The listing builds one solid part. Answer for the finished solid, in the listing's coordinates (mm). Coordinates: 2 decimals unless noted, no trailing zeros. Order: outer loops, then holes, each group sorted by start corner. A loop starts at its lowest first (then second) coordinate and runs counter-clockwise, first axis right, second up. Notation, with made-up numbers: (-23, 3) - (7, 3) arc R16 ccw to (7, 28) - close; hole circle Ø7 at (11.25, 28.25). An arc over 180 degrees is marked (long way). One line per item, written item: value. Start each with the question number.
```python
from build123d import *

# Parameters (mm, degrees)
BOSS_EXTRUDE1_DEPTH             = 16
SKETCH2_W                       = 34
SKETCH2_H                       = 8
CUT_EXTRUDE1_DEPTH              = 0.5
SKETCH7_R                       = 8.5
CUT_EXTRUDE2_DEPTH              = 2
BOSS_EXTRUDE2_DEPTH             = 3
BOSS_EXTRUDE3_REACH             = 31.159
BOSS_EXTRUDE3_DIRECTION_2_REACH = 31.159
SKETCH11_W                      = 2.65
SKETCH11_H                      = 24
M5_CLEARANCE_HOLE2_AT_2_COUNT   = 2
M5_CLEARANCE_HOLE2_AT_2_PITCH   = 25.394250395
M5_CLEARANCE_HOLE2_AT_3_COUNT   = 2
M5_CLEARANCE_HOLE2_AT_3_PITCH   = 19.596880573
M5_CLEARANCE_HOLE2_AT_4_COUNT   = 2
M5_CLEARANCE_HOLE2_AT_4_PITCH   = 14.465476141
MOVE_FACE1_BY                   = 0.5
FILLET1_R                       = 0.4
CHAMFER1_SIZE                   = 0.6
FILLET2_R                       = 0.2


# Read off the part's stored shape, not the designer's step: M4 Tapped Hole2
with BuildPart() as part:
    # Sketch1 → Boss-Extrude1 (new body)
    with BuildSketch(Plane(origin=(0, -16.5, 0), x_dir=(-1, 0, 0), z_dir=(0, -1, 0))):
        with BuildLine():
            Line((17, -17), (-17, -17))
            Line((-17, -17), (-17, 0))
            ThreePointArc((-17, 0), (0, 17), (17, 0))
            Line((17, 0), (17, -17))
        make_face()
    extrude(amount=-BOSS_EXTRUDE1_DEPTH)

    # Sketch2 → Cut-Extrude1 (cut)
    with BuildSketch(Plane(origin=(0, -0.5, 0), x_dir=(1, 0, 0), z_dir=(0, 1, 0))):
        with Locations((0, -10.5)):
            Rectangle(SKETCH2_W, SKETCH2_H)
    extrude(amount=-CUT_EXTRUDE1_DEPTH, mode=Mode.SUBTRACT)

    # Sketch7 → Cut-Extrude2 (cut)
    with BuildSketch(Plane.XZ.offset(16.5)):
        with Locations(Location((0, 0, 0), (0, 0, 270))):
            Circle(SKETCH7_R)
    extrude(amount=-CUT_EXTRUDE2_DEPTH, mode=Mode.SUBTRACT)

    # Sketch8 → Boss-Extrude2 (add)
    with BuildSketch(Plane(origin=(0, -0.5, 0), x_dir=(1, 0, 0), z_dir=(0, 1, 0))):
        with BuildLine():
            Line((-17, -4), (17, -4))
            Line((17, -4), (17, 0))
            ThreePointArc((17, 0), (0, 17), (-17, 0))
            Line((-17, 0), (-17, -4))
        make_face()
    extrude(amount=BOSS_EXTRUDE2_DEPTH)


with BuildPart() as body_2:

    # Boss-Extrude3: up to this face of the body (flat: up to its plane)
    boss_extrude3_end = Plane(part.part.faces().sort_by_distance((17, -8.203571429, 8.192857143))[0])
    # Sketch9 → Boss-Extrude3 (new, up to the picked face)
    with BuildSketch(Plane(origin=(0, 0, 0), x_dir=(0, 0, -1), z_dir=(1, 0, 0)), mode=Mode.PRIVATE) as boss_extrude3_sk1:
        Polygon((-14.5, 1), (-14.5, 0.5), (-17, 0.5), (-17, 7.5), (-4, 7.5), (-4, 0.5), (-6.5, 0.5), (-6.5, 1), align=None)
    boss_extrude3_tool1 = split(extrude(boss_extrude3_sk1.sketch, amount=BOSS_EXTRUDE3_REACH, mode=Mode.PRIVATE), bisect_by=boss_extrude3_end, keep=Keep.BOTH, mode=Mode.PRIVATE)
    add(boss_extrude3_tool1.solids().sort_by(Axis((0, 4.149425, 10.5), (1, 0, 0)))[0])


    # Boss-Extrude3 direction 2: up to this face of the body (flat: up to its plane)
    boss_extrude3_direction_2_end = Plane(part.part.faces().sort_by_distance((-17, -8.203571429, 8.192857143))[0])
    # Sketch9 → Boss-Extrude3 direction 2 (add, up to the picked face)
    with BuildSketch(Plane(origin=(0, 0, 0), x_dir=(0, 0, -1), z_dir=(1, 0, 0)), mode=Mode.PRIVATE) as boss_extrude3_direction_2_sk1:
        Polygon((-14.5, 1), (-14.5, 0.5), (-17, 0.5), (-17, 7.5), (-4, 7.5), (-4, 0.5), (-6.5, 0.5), (-6.5, 1), align=None)
    boss_extrude3_direction_2_tool1 = split(extrude(boss_extrude3_direction_2_sk1.sketch, amount=-BOSS_EXTRUDE3_DIRECTION_2_REACH, mode=Mode.PRIVATE), bisect_by=boss_extrude3_direction_2_end, keep=Keep.BOTH, mode=Mode.PRIVATE)
    add(boss_extrude3_direction_2_tool1.solids().sort_by(Axis((0, 4.149425, 10.5), (-1, 0, 0)))[0])


with BuildPart() as m5_clearance_hole2_tool:
    # Sketch11 → M5 Clearance Hole2 (revolve)
    with BuildSketch(Plane(origin=(7.232738071, 7.5, 10.5), x_dir=(0, 0, 1), z_dir=(1, 0, 0))):
        with Locations((1.325, 12)):
            Rectangle(SKETCH11_W, SKETCH11_H)
    m5_clearance_hole2 = revolve(axis=Axis((7.232738071, 13.85, 10.5), (0, -1, 0)))


with BuildPart() as part_1:
    add(part.part)

    # M5 Clearance Hole2: cut by m5_clearance_hole2_tool
    add(m5_clearance_hole2_tool.part, mode=Mode.SUBTRACT)

    # M5 Clearance Hole2 at 2: M5 Clearance Hole2 ×2
    with Locations(*[Vector(-0.6398436369623559, 0, -0.768505120502645) * (i * M5_CLEARANCE_HOLE2_AT_2_PITCH) for i in range(1, M5_CLEARANCE_HOLE2_AT_2_COUNT)]):
        add(m5_clearance_hole2, mode=Mode.SUBTRACT)

    # M5 Clearance Hole2 at 3: M5 Clearance Hole2 ×2
    with Locations(*[Vector(0.09097740748886189, 0, -0.9958529566791503) * (i * M5_CLEARANCE_HOLE2_AT_3_PITCH) for i in range(1, M5_CLEARANCE_HOLE2_AT_3_COUNT)]):
        add(m5_clearance_hole2, mode=Mode.SUBTRACT)


with BuildPart() as body_2_1:
    add(body_2.part)

    # M5 Clearance Hole2: cut by m5_clearance_hole2_tool
    add(m5_clearance_hole2_tool.part, mode=Mode.SUBTRACT)


with BuildPart() as m5_clearance_hole2_at_4_tool:
    # M5 Clearance Hole2 at 4: M5 Clearance Hole2 ×2
    with Locations(*[(-i * M5_CLEARANCE_HOLE2_AT_4_PITCH, 0, 0) for i in range(1, M5_CLEARANCE_HOLE2_AT_4_COUNT)]):
        add(m5_clearance_hole2)


with BuildPart() as part_2:
    add(part_1.part)

    # M5 Clearance Hole2 at 4: cut by m5_clearance_hole2_at_4_tool
    add(m5_clearance_hole2_at_4_tool.part, mode=Mode.SUBTRACT)

    # M4 Tapped Hole2 outline → M4 Tapped Hole2 (revolve, cut)
    with BuildSketch(Plane(origin=(0, -3.5, 5), x_dir=(0, 1, 0), z_dir=(0, 0, -1))):
        Polygon((0, 17), (0, 5.908579979), (1.65, 6.9), (1.65, 17), align=None)
        Polygon((1.65, -6.9), (0, -5.908579979), (0, -17), (1.65, -17), align=None)
    revolve(axis=Axis((0, -3.5, 5), (1, 0, 0)), mode=Mode.SUBTRACT)

    # M4 Tapped Hole2 2 outline → M4 Tapped Hole2 2 (revolve, cut)
    with BuildSketch(Plane(origin=(0, -11.5, 5), x_dir=(0, 1, 0), z_dir=(0, 0, -1))):
        Polygon((0, 17), (0, 5.908579979), (1.65, 6.9), (1.65, 17), align=None)
        Polygon((1.65, -6.9), (0, -5.908579979), (0, -17), (1.65, -17), align=None)
    revolve(axis=Axis((0, -11.5, 5), (1, 0, 0)), mode=Mode.SUBTRACT)

    # Move Face1: a face moved inward by 0.5
    extrude(part_2.faces().sort_by_distance((0, -14.5, 0))[0], amount=MOVE_FACE1_BY, dir=(0, 1, 0), mode=Mode.SUBTRACT)

    # Fillet1
    fillet1_edges = [part_2.edges().sort_by_distance(p)[0] for p in [
        (0, -14, 8.5),
    ]]
    fillet(fillet1_edges, radius=FILLET1_R)

    # Chamfer1
    chamfer1_edges = [part_2.edges().sort_by_distance(p)[0] for p in [
        (0, -16.5, 8.5),
    ]]
    chamfer(chamfer1_edges, length=CHAMFER1_SIZE)

    # Fillet2
    fillet2_edges = [part_2.edges().sort_by_distance(p)[0] for p in [
        (0, -0.5, 4),
    ]]
    fillet(fillet2_edges, radius=FILLET2_R)


with BuildPart() as body_2_2:
    add(body_2_1.part)

    # M5 Clearance Hole2 at 4: cut by m5_clearance_hole2_at_4_tool
    add(m5_clearance_hole2_at_4_tool.part, mode=Mode.SUBTRACT)


solid = body_2_2.part
```
(1) For a pull along Z with two mould halves and no side action, classify faces 1 (the face through (0, 1, 10)), 2 (the face through (0, 4, 17)), 3 (the face through (0, 0.5, 16)) as pulls with the +Z half, pulls with the -Z half, needs draft (parallel to the pull), parting line crosses it, or undercut.
(2) Consider probe 1 along X at (y, z) = (4.5, 10.5); probe 2 along Y at (x, z) = (13, 9.5); probe 3 along Z at (x, y) = (9, 1.5). Determine where each line is inside the solid, lowest interval first.
(3) The part is cut by section C-C on y = 6. Determine the outline of the cut face in (x, z).
(4) A flat-ended cylindrical pin translates along its axis: pin 1 Ø4 at (x, z) = (3, 11) entering from -Y. Find the tip coordinate at first contact, or state that the pin passes through.
(5) The part is cut by section D-D on x = 6.5. Determine the outline of the cut face in (y, z), plus the area to 3 significant figures.
(6) The part is cut by section B-B on x = 12. Determine the outline of the cut face in (y, z).
(7) The part is cut by section A-A on z = 8.5. Determine the outline of the cut face in (x, y).
Completed:
1. face 1: undercut
1. face 2: pulls with the +Z half
1. face 3: needs draft
2. probe 1: x = -17 to -9.88, -4.58 to 4.58, 9.88 to 17
2. probe 2: y = 1 to 7.5
2. probe 3: z = 4 to 8.53, 12.47 to 17
3. outline: (-17, 4) - (17, 4) - (17, 17) - (-17, 17) - close; hole circle Ø5.3 at (-7.23, 10.5); hole circle Ø5.3 at (7.23, 10.5)
4. pin 1: stops at y = 1
5. outline: (0.5, 4) - (7.5, 4) - (7.5, 7.95) - (1, 7.95) - (1, 6.5) - (0.5, 6.5) - close; (0.5, 14.5) - (1, 14.5) - (1, 13.05) - (7.5, 13.05) - (7.5, 17) - (0.5, 17) - close
5. area: 53.9 mm2
6. outline: (0.5, 4) - (7.5, 4) - (7.5, 17) - (0.5, 17) - (0.5, 14.5) - (1, 14.5) - (1, 6.5) - (0.5, 6.5) - close
7. outline: (-17, 1) - (-8.97, 1) - (-8.97, 7.5) - (-17, 7.5) - close; (-5.49, 1) - (5.49, 1) - (5.49, 7.5) - (-5.49, 7.5) - close; (8.97, 1) - (17, 1) - (17, 7.5) - (8.97, 7.5) - close
